from build123d import *

# Parameters (mm, degrees)
F0_R      = 25
F1_DEPTH  = 4
F3_R      = 27
F4_DEPTH  = 4.4
F5_DEPTH  = 14.5
F6_R      = 27
F6_R_2    = 25.1
F7_DEPTH  = 15
F9_R      = 3
F10_SIZE  = 1
F11_R     = 3
F12_DEPTH = 3


# Not quite as in the source:
# - a fillet or chamfer that OpenCascade refuses, or shapes differently, is made with other operations: its cross-section is extruded or revolved along the edge and cut away or added
# - a feature names something its author has since deleted; it is built from what else it names


with BuildPart() as f1:
    # F0 (on Top) → F1 (new body)
    with BuildSketch(Plane.XY):
        Circle(F0_R)
    extrude(amount=F1_DEPTH)

    # F3 (on face) → F4 (join)
    with BuildSketch(Plane(origin=(0, 0, 0), x_dir=(1, 0, 0), z_dir=(0, 0, -1))):
        Circle(F3_R)
    extrude(amount=-F4_DEPTH)

    # F2 (on face) → F5 (join)
    with BuildSketch(Plane.XY.offset(4)):
        Polygon((1.8290777225, -14.20661062), (0, -13.8), (-1.8290777225, -14.20661062), (-1.8290777225, -16.5130756795), (0, -17.6663082093), (1.8290777225, -16.5130756795), align=None)
        Polygon((10.7892744581, -8.6041592657), (9.9667641351, -10.2877073879), (11.7700311319, -11.7257648309), (13.812075937, -11.014763005), (14.0508537454, -8.8657037362), (12.2475867487, -7.4276462932), align=None)
        Polygon((13.4540051881, 3.0707888886), (14.257429314, 1.3780493383), (16.506066479, 1.8912860975), (17.2233769785, 3.9311234023), (15.6920503129, 5.4577239479), (13.4434131479, 4.9444871887), align=None)
        Polygon((5.9875955998, 12.4333703771), (7.811959421, 12.0061068057), (8.8126971051, 14.0841600192), (7.6651238623, 15.9167937073), (5.5168129352, 15.671374182), (4.5160752511, 13.5933209684), align=None)
        Polygon((-5.9875955998, 12.4333703771), (-4.5160752511, 13.5933209684), (-5.5168129352, 15.671374182), (-7.6651238623, 15.9167937073), (-8.8126971051, 14.0841600192), (-7.811959421, 12.0061068057), align=None)
        Polygon((-13.4540051881, 3.0707888886), (-13.4434131479, 4.9444871887), (-15.6920503129, 5.4577239479), (-17.2233769785, 3.9311234023), (-16.506066479, 1.8912860975), (-14.257429314, 1.3780493383), align=None)
        Polygon((-10.7892744581, -8.6041592657), (-12.2475867487, -7.4276462932), (-14.0508537454, -8.8657037362), (-13.812075937, -11.014763005), (-11.7700311319, -11.7257648309), (-9.9667641351, -10.2877073879), align=None)
        Polygon((2.2625249746, -5.6745974369), (0, -4.5038154349), (-2.2625249746, -5.6745974369), (0, -7.3385047726), align=None)
        Polygon((3.7830830493, 4.7967028232), (3.9004185806, 2.2519077174), (6.0456080239, 0.8778946137), (6.3553315589, 3.6692523863), align=None)
        Polygon((-6.0456080239, 0.8778946137), (-3.9004185806, 2.2519077174), (-3.7830830493, 4.7967028232), (-6.3553315589, 3.6692523863), align=None)
    extrude(amount=F5_DEPTH)

    # F6 (on face) → F7 (join)
    with BuildSketch(Plane.XY.offset(4.4)):
        Circle(F6_R)
        Circle(F6_R_2, mode=Mode.SUBTRACT)
    extrude(amount=F7_DEPTH)

    # F8: fillet of radius 2 on 1 edges, made by hand

    # F8_s1 → F8_t2 (revolve, cut)
    with BuildSketch(Plane.XZ):
        with BuildLine():
            ThreePointArc((27, 17.4025015645), (26.4491376746, 18.7809064397), (25.1, 19.4))
            Line((25.1, 19.4), (27, 19.4))
            Line((27, 19.4), (27, 17.4025015645))
        make_face()
    revolve(axis=Axis((0, 0, 19.4), (0, 0, 1)), mode=Mode.SUBTRACT)

    # F9
    f9_edges = [f1.edges().sort_by_distance(p)[0] for p in [
        (-27, 0, 0),
    ]]
    fillet(f9_edges, radius=F9_R)

    # F10
    f10_edges = [f1.edges().sort_by_distance(p)[0] for p in [
        (1.131262, -5.089206, 18.5),
        (-1.131262, -5.089206, 18.5),
        (-1.131262, -6.506551, 18.5),
        (1.131262, -6.506551, 18.5),
        (6.20047, 2.273574, 18.5),
        (5.069207, 4.232978, 18.5),
        (3.841751, 3.524305, 18.5),
        (4.973013, 1.564901, 18.5),
        (5.016444, 14.632348, 18.5),
        (5.251835, 13.013346, 18.5),
        (6.899778, 12.219739, 18.5),
        (8.312328, 13.045133, 18.5),
        (8.23891, 15.000477, 18.5),
        (6.590968, 15.794084, 18.5),
        (-5.069207, 4.232978, 18.5),
        (-6.20047, 2.273574, 18.5),
        (-4.973013, 1.564901, 18.5),
        (-3.841751, 3.524305, 18.5),
        (-5.251835, 13.013346, 18.5),
        (-5.016444, 14.632348, 18.5),
        (-6.590968, 15.794084, 18.5),
        (-8.23891, 15.000477, 18.5),
        (-8.312328, 13.045133, 18.5),
        (-6.899778, 12.219739, 18.5),
        (13.855717, 2.224419, 18.5),
        (15.381748, 1.634668, 18.5),
        (16.864722, 2.911205, 18.5),
        (16.457714, 4.694424, 18.5),
        (14.567732, 5.201106, 18.5),
        (13.448709, 4.007638, 18.5),
        (10.378019, -9.445933, 18.5),
        (10.868398, -11.006736, 18.5),
        (12.791054, -11.370264, 18.5),
        (13.931465, -9.940233, 18.5),
        (13.14922, -8.146675, 18.5),
        (11.518431, -8.015903, 18.5),
        (0.914539, -14.003305, 18.5),
        (-0.914539, -14.003305, 18.5),
        (-1.829078, -15.359843, 18.5),
        (-0.914539, -17.089692, 18.5),
        (0.914539, -17.089692, 18.5),
        (1.829078, -15.359843, 18.5),
        (-11.518431, -8.015903, 18.5),
        (-13.14922, -8.146675, 18.5),
        (-13.931465, -9.940233, 18.5),
        (-12.791054, -11.370264, 18.5),
        (-10.868398, -11.006736, 18.5),
        (-10.378019, -9.445933, 18.5),
        (-15.381748, 1.634668, 18.5),
        (-13.855717, 2.224419, 18.5),
        (-13.448709, 4.007638, 18.5),
        (-14.567732, 5.201106, 18.5),
        (-16.457714, 4.694424, 18.5),
        (-16.864722, 2.911205, 18.5),
    ]]
    chamfer(f10_edges, length=F10_SIZE)

    # F11 (on face) → F12 (cut)
    with BuildSketch(Plane.XY.offset(4.4)):
        Circle(F11_R)
    extrude(amount=-F12_DEPTH, mode=Mode.SUBTRACT)


solid = f1.part
Input: part model. Units: mm. Frame: model coordinates. Coordinates: 2 decimals unless noted, no trailing zeros. Order: outer loops, then holes, each group sorted by start corner. A loop starts at its lowest first (then second) coordinate and runs counter-clockwise, first axis right, second up. Notation, with made-up numbers: M -7.75,-38 L 13.25,-38 A12 cw 13.25,-17 Z; hole C 21,-2 d11. An arc over 180 degrees is marked long. Write item = value, one per line. Start each with the question number.
(1) Line query: line 1 along Y through (x, z) = (0, 16.25); line 2 along X through (y, z) = (-14.5, 6); line 3 along Y through (x, z) = (0, 3.1). Output: solid intervals per line, ascending. Write a range as [from, to].
(2) Pull-direction query (X, two-part tool) for faces 1 (the flat face through (-12.89, -8.45, 17.9)), 2 (the flat face through (-7.96, 13.23, 17.9)); classes: released by +X, released by -X, zero draft, split by the parting line, or undercut.
(3) Section B-B on z = 12.75. Give the number of separate pieces and of enclosed holes in the cut face, and give its area (3 significant figures).
(4) Section A-A on y = 0. Output: boundary loops of the cut face in (x, z).
(5) First-contact query: P1, Ø10, axis at y = 10, z = 17, coming from the -X side; P2, Ø0.5, axis at x = -7, y = 14, coming from the +Z side; P3, Ø1.8, axis at x = -1, y = -1.5, coming from the +Z side. Flat tips, straight axial feed; report the tip coordinate or a pass-through.
Result set:
q1.line_1 = [-27, -25.1], [-17.67, -13.8], [-7.34, -4.5], [25.1, 27]
q1.line_2 = [-22.78, -20.49], [-1.83, 1.83], [20.49, 22.78]
q1.line_3 = [-27, -3], [3, 27]
q2.face_1 = undercut
q2.face_2 = undercut
q3.separate_pieces = 11
q3.enclosed_holes = 1
q3.area = 409 mm²
q4.outline = M -27,3 A3 ccw -24,0 L 24,0 A3 ccw 27,3 L 27,17.4 A2 ccw 25.1,19.4 L 25.1,4.4 L 3,4.4 L 3,1.4 L -3,1.4 L -3,4.4 L -25.1,4.4 L -25.1,19.4 A2 ccw -27,17.4 Z
q5.P1 = -26.53
q5.P2 = 18.5
q5.P3 = 1.4
